Source: CAD feature listing. Evaluate the final solid. Frame: model axes, mm. A direction names the side the tool comes from. Give positions to 0.01 mm unless a question says otherwise; leave off trailing zeros. Order: outer loops, then holes, each group sorted by start corner. A loop starts at its lowest first (then second) coordinate and runs counter-clockwise, first axis right, second up. Notation, with made-up numbers: M 0,57 L 45,57 A14 ccw 45,63 Z; hole C 77.5,-1.75 d9. An arc over 180 degrees is marked long. Answer in a Markdown table with one row per item. Add a question column.
(1) Section query A-A, the plane x = 0. Return loops of the section in (y, z), plus the area to 3 significant figures.
(2) Section query C-C, the plane y = 37. Return loops of the section in (x, z), plus the area to 3 significant figures.
(3) Material intervals for line 1 along Z through (x, y) = (0, 2.9); line 2 along Z through (x, y) = (0, 39.25), sorted ascending.
(4) Pin query (flat end, axial travel): P1, Ø1, axis at y = 17.5, z = -4.5, coming from the -X side; P2, Ø5.5, axis at x = 0, z = 0, coming from the -Y side; P3, Ø2, axis at x = 1.5, y = 13, coming from the +Z side. Return the tip coordinate at first contact, or that it passes through.
(5) Section query B-B, the plane z = 0. Return loops of the section in (x, y), plus the area to 3 significant figures.
(6) Mould query, pull axis X, two halves, no side actions, for faces 1 (the face through (-6, 2, 0)), 2 (the face through (0, 34, 0)), 3 (the face through (3.233, 1.972, -1.341)), 4 (the face through (3, 0, 3)). Classes: pulls with the +X half, pulls with the -X half, needs draft (parallel to the pull), parting line crosses it, or undercut.
(7) Section query D-D, the plane y = 10.5. Return loops of the section in (x, z), plus the area to 3 significant figures.
(8) Set-up query: faces 5 (the face through (-6, 39, 0)), 6 (the face through (2, 44, 6)), 7 (the face through (2, 4, 6)). Return all of +Z, -Z, +X, -X, +Y, -Y with unobstructed straight access to the full face (end or side cutting, diameter ignored); none if empty.
from build123d import *

# Parameters (mm, degrees)
SKETCH1_R           = 6
BOSS_EXTRUDE1_DEPTH = 4
SKETCH2_R           = 9
BOSS_EXTRUDE2_DEPTH = 40
SKETCH3_R           = 3.5
CUT_EXTRUDE1_DEPTH  = 4
SKETCH4_R           = 6
CUT_EXTRUDE2_DEPTH  = 10


with BuildPart() as part:
    # Sketch1 → Boss-Extrude1 (new body)
    with BuildSketch(Plane(origin=(0, 0, 0), x_dir=(1, 0, 0), z_dir=(0, 1, 0))):
        Circle(SKETCH1_R)
    extrude(amount=BOSS_EXTRUDE1_DEPTH)

    # Sketch2 → Boss-Extrude2 (add)
    with BuildSketch(Plane(origin=(0, 4, 0), x_dir=(1, 0, 0), z_dir=(0, 1, 0))):
        Circle(SKETCH2_R)
    extrude(amount=BOSS_EXTRUDE2_DEPTH)

    # Sketch3 → Cut-Extrude1 (cut)
    with BuildSketch(Plane.XZ):
        Circle(SKETCH3_R)
    extrude(amount=-CUT_EXTRUDE1_DEPTH, mode=Mode.SUBTRACT)

    # Sketch4 → Cut-Extrude2 (cut)
    with BuildSketch(Plane(origin=(0, 44, 0), x_dir=(1, 0, 0), z_dir=(0, 1, 0))):
        Circle(SKETCH4_R)
    extrude(amount=-CUT_EXTRUDE2_DEPTH, mode=Mode.SUBTRACT)


solid = part.part
Values follow:
| question | item | result |
|---|---|---|
| 1 | outline | M 0,-6 L 4,-6 L 4,-9 L 44,-9 L 44,-6 L 34,-6 L 34,6 L 44,6 L 44,9 L 4,9 L 4,6 L 0,6 L 0,3.5 L 4,3.5 L 4,-3.5 L 0,-3.5 Z |
| 1 | area | 620 mm² |
| 2 | outline | C 0,0 d18; hole C 0,0 d12 |
| 2 | area | 141 mm² |
| 3 | line 1 | z = -6 to -3.5, 3.5 to 6 |
| 3 | line 2 | z = -9 to -6, 6 to 9 |
| 4 | P1 | stops at x = -8.06 |
| 4 | P2 | stops at y = 4 |
| 4 | P3 | stops at z = 8.99 |
| 5 | outline | M -9,4 L -6,4 L -6,0 L -3.5,0 L -3.5,4 L 3.5,4 L 3.5,0 L 6,0 L 6,4 L 9,4 L 9,44 L 6,44 L 6,34 L -6,34 L -6,44 L -9,44 Z |
| 5 | area | 620 mm² |
| 6 | face 1 | parting line crosses it |
| 6 | face 2 | undercut |
| 6 | face 3 | undercut |
| 6 | face 4 | needs draft |
| 7 | outline | C 0,0 d18 |
| 7 | area | 254 mm² |
| 8 | face 5 | +Y |
| 8 | face 6 | +Z, -Z, +X, -X, +Y |
| 8 | face 7 | -Y |
